Geometry check sheet. Reference: the model listing, model coordinates, mm. A direction names the side the tool comes from. Give positions to 0.01 mm unless a question says otherwise; leave off trailing zeros. Loops run counter-clockwise (first coordinate to the right, second up) from the corner with the lowest first, then second, coordinate; pieces in that order, holes last. Notation, with made-up numbers: (35, 0) -> (57, 0) arc R18 ccw to (57, 15) -> close; hole circle Ø4 at (12.5, -22.75). An arc over 180 degrees is marked (long way). Answer in a Markdown table with one row per item. Add a question column.
Autodesk Inventor part; units mm, degrees
ref_plane "YZ Plane" through (0, 0, 0) normal (1, 0, 0) x (0, 1, 0)
ref_plane "XZ Plane" through (0, 0, 0) normal (0, 1, 0) x (-1, 0, 0)
ref_plane "XY Plane" through (0, 0, 0) normal (0, 0, 1) x (1, 0, 0)
sketch "Sketch1" plane through (0, 0, 0) normal (0, 0, 1) x (1, 0, 0)
  line L0 (-58.4998, -9.3705) -> (144.5002, -9.3705)
  line L1 (144.5002, -9.3705) -> (144.5002, -119.3705)
  line L2 (144.5002, -119.3705) -> (-58.4998, -119.3705)
  line L3 (-58.4998, -119.3705) -> (-58.4998, -9.3705)
  line L4 (-58.4998, -9.3705) -> (-38.4998, -9.3705)
  line L5 (-38.4998, -9.3705) -> (-38.4998, -21.3705)
  line L6 (-38.4998, -21.3705) -> (-58.4998, -21.3705)
  line L7 (-58.4998, -21.3705) -> (-58.4998, -9.3705)
  line L8 (144.5002, -9.3705) -> (124.5002, -9.3705)
  line L9 (124.5002, -9.3705) -> (124.5002, -21.3705)
  line L10 (124.5002, -21.3705) -> (144.5002, -21.3705)
  line L11 (144.5002, -21.3705) -> (144.5002, -9.3705)
  circle A0 centre (-56.009, -27.3705) radius 2
  circle A1 centre (142.0094, -27.3705) radius 2
  circle A2 centre (43.0002, -17.3705) radius 2
  circle A3 centre (-56.009, -111.8705) radius 2
  circle A4 centre (42.0002, -111.8705) radius 2
  circle A5 centre (142.0094, -113.8705) radius 2
  point P0 (0, 0)
  dimension "d0" = 203
  dimension "d1" = 110
  dimension "d2" = 20
  dimension "d3" = 12
  dimension "d4" = 20
  dimension "d5" = 12
  dimension "d6" = 4
  dimension "d7" = 4
  dimension "d8" = 198.0184
  dimension "d9" = 2.4908
  dimension "d10" = 18
  dimension "d11" = 4
  dimension "d12" = 10
  dimension "d13" = 99.0092
  dimension "d14" = 4
  dimension "d15" = 84.5
  dimension "d16" = 4
  dimension "d17" = 4
  dimension "d18" = 0
extrude "Extrusion1" add sketch "Sketch1" along normal blind 2 contours L0 L9 L10 L1 L2 L3 L6 L5
sketch "Sketch2" plane through (0, 0, 2) normal (0, 0, 1) x (1, 0, 0)
  circle A0 centre (134.5002, -99.3705) radius 1.5
  line L0 (144.5002, -119.3705) -> (144.5002, -21.3705)
  line L1 (-58.4998, -119.3705) -> (144.5002, -119.3705)
  circle A1 centre (134.5002, -32.6905) radius 1.5
  circle A2 centre (88.7802, -99.3705) radius 1.5
  circle A3 centre (88.7802, -32.6905) radius 1.5
  circle A4 centre (68.7802, -99.3705) radius 1.5
  circle A5 centre (68.7802, -32.6905) radius 1.5
  circle A6 centre (23.0602, -32.6905) radius 1.5
  circle A7 centre (23.0602, -99.3705) radius 1.5
  circle A8 centre (-44.9398, -59.5668) radius 2
  circle A9 centre (3.0602, -59.5668) radius 2
  point P0 (0, 0)
  dimension "d21" = 3
  dimension "d22" = 10
  dimension "d23" = 20
  dimension "d24" = 3
  dimension "d25" = 10
  dimension "d26" = 66.68
  dimension "d27" = 3
  dimension "d28" = 45.72
  dimension "d29" = 3
  dimension "d30" = 45.72
  dimension "d31" = 66.68
  dimension "d32" = 3
  dimension "d33" = 20
  dimension "d34" = 3
  dimension "d35" = 3
  dimension "d36" = 45.72
  dimension "d37" = 20
  dimension "d38" = 3
  dimension "d39" = 4
  dimension "d40" = 4
  dimension "d41" = 48
  dimension "d42" = 20
extrude "Extrusion2" cut sketch "Sketch2" against normal blind 2
sketch "Sketch3" plane through (0, 0, 0) normal (0, 0, -1) x (-1, 0, 0)
  circle A0 centre (56.009, -111.8705) radius 2
  circle A1 centre (-42.0002, -111.8705) radius 2
  circle A2 centre (-142.0094, -113.8705) radius 2
  circle A3 centre (-142.0094, -27.3705) radius 2
  circle A4 centre (-43.0002, -17.3705) radius 2
  circle A5 centre (56.009, -27.3705) radius 2
  circle A6 centre (56.009, -111.8705) radius 6
  circle A7 centre (-42.0002, -111.8705) radius 6
  circle A8 centre (-142.0094, -113.8705) radius 2
  circle A9 centre (-142.0094, -113.8705) radius 6
  circle A10 centre (-43.0002, -17.3705) radius 6
  circle A11 centre (-142.0094, -27.3705) radius 6
  circle A12 centre (56.009, -27.3705) radius 6
  circle A13 centre (56.009, -111.8705) radius 4
  circle A14 centre (-42.0002, -111.8705) radius 4
  circle A15 centre (56.009, -27.3705) radius 4
  circle A16 centre (-43.0002, -17.3705) radius 4
  circle A17 centre (-142.0094, -27.3705) radius 4
  circle A18 centre (-142.0094, -113.8705) radius 4
  point P0 (0, 0)
  dimension "d45" = 12
  dimension "d46" = 12
  dimension "d47" = 12
  dimension "d48" = 12
  dimension "d49" = 12
  dimension "d50" = 12
  dimension "d51" = 8
  dimension "d52" = 8
  dimension "d53" = 8
  dimension "d54" = 8
  dimension "d55" = 8
  dimension "d56" = 8
extrude "Extrusion3" add sketch "Sketch3" along normal blind 3 contours A6 | A7 | A9 | A10 | A11 | A12
sketch "Sketch4" plane through (0, 0, 2) normal (0, 0, 1) x (1, 0, 0)
  line L0 (124.5002, -9.3705) -> (-38.4998, -9.3705)
  line L1 (-38.4998, -9.3705) -> (-38.4998, -21.3705)
  line L2 (-38.4998, -21.3705) -> (-58.4998, -21.3705)
  line L3 (-58.4998, -21.3705) -> (-58.4998, -119.3705)
  line L4 (-58.4998, -119.3705) -> (144.5002, -119.3705)
  line L5 (144.5002, -119.3705) -> (144.5002, -21.3705)
  line L6 (144.5002, -21.3705) -> (124.5002, -21.3705)
  line L7 (124.5002, -21.3705) -> (124.5002, -9.3705)
  line L8 (-77.131, 13.4165) -> (211.8208, 13.4165)
  line L9 (211.8208, 13.4165) -> (211.8208, -174.2275)
  line L10 (211.8208, -174.2275) -> (-77.131, -174.2275)
  line L11 (-77.131, -174.2275) -> (-77.131, 13.4165)
  point P0 (0, 0)
extrude "Extrusion4" cut sketch "Sketch4" against normal through all
equation "\"d13\" = 0.5 * d8"
properties part number "RoboClawPlate"
1. Sectioned sample at A-A (z = -1.4). Enter the section's corners in (x, y), plus the area to 3 significant figures.
2. Gauge pin test, flat ends, axial feed: pin 1 Ø1 at (x, z) = (136, 0.5) entering from +Y; pin 2 Ø5 at (x, y) = (51, -68) entering from -Z; pin 3 Ø1 at (y, z) = (-13, 0.5) entering from -X. Record the tip position at first contact, or that the pin passes through.
3. Release check for a two-part mould opening along X. For faces 1 (the face through (-58.5, -71, 1)), 2 (the face through (-51, -27, -3)), 3 (the face through (42.78, -117.82, -1.48)) record: released by +X, released by -X, zero draft, split by the parting line, or undercut.
4. Access from +Z, -Z, +X, -X, +Y, -Y to the whole of each face (thin tool, end or side, straight path). Record for faces 4 (the face through (-51, -112, -3)), 5 (the face through (139.8, -27.3, 0)).
5. Material ranges on L1, parallel to Y at x = 43.5, z = 0.05; L2, parallel to X at y = -17, z = -2.65; L3, parallel to Z at x = 6.5, y = -74.5, recorded low to high. Write a range as from..to.
6. Sectioned sample at C-C (y = -72.5). Enter the section's corners in (x, z), plus the area to 3 significant figures.
7. Sectioned sample at B-B (x = 129). Enter the section's corners in (y, z), plus the area to 3 significant figures.
Response:
| question | item | result |
|---|---|---|
| 1 | outline | (-58.5, -117.33) arc R6 ccw (long way) to (-58.5, -106.41) -> (-58.5, -108.74) arc R4 cw (long way) to (-58.5, -115) -> close; (-58.5, -32.83) arc R6 ccw (long way) to (-58.5, -21.91) -> (-58.5, -24.24) arc R4 cw (long way) to (-58.5, -30.5) -> close; circle Ø12 at (42, -111.87); circle Ø12 at (43, -17.37); (139.61, -119.37) -> (144.41, -119.37) arc R6 ccw to (144.5, -119.33) -> (144.5, -117) arc R4 cw (long way) to (144.5, -110.74) -> (144.5, -108.41) arc R6 ccw (long way) to start; (144.5, -32.83) -> (144.5, -30.5) arc R4 cw (long way) to (144.5, -24.24) -> (144.5, -21.91) arc R6 ccw (long way) to start; hole circle Ø8 at (42, -111.87); hole circle Ø8 at (43, -17.37) |
| 1 | area | 292 mm2 |
| 2 | pin 1 | stops at y = -21.37 |
| 2 | pin 2 | stops at z = 0 |
| 2 | pin 3 | stops at x = -38.5 |
| 3 | face 1 | released by -X |
| 3 | face 2 | zero draft |
| 3 | face 3 | undercut |
| 4 | face 4 | -Z, +X, -X, +Y, -Y |
| 4 | face 5 | -Z |
| 5 | L1 | y = -119.37..-113.19, -110.55..-19.31, -15.43..-9.37 |
| 5 | L2 | x = 37.01..39.02, 46.98..48.99 |
| 5 | L3 | z = 0..2 |
| 6 | outline | (-58.5, 0) -> (144.5, 0) -> (144.5, 2) -> (-58.5, 2) -> close |
| 6 | area | 406 mm2 |
| 7 | outline | (-119.37, 0) -> (-21.37, 0) -> (-21.37, 2) -> (-119.37, 2) -> close |
| 7 | area | 196 mm2 |
